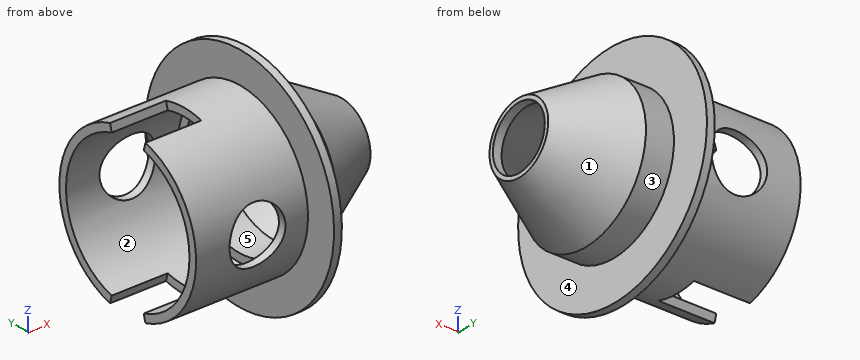
from build123d import *

# Parameters (mm, degrees)
F3_DEPTH = 6.35
F5_D     = 6.35
F6_D     = 6.35


with BuildPart() as f1:
    # F0 (on Front) → F1 (revolve)
    with BuildSketch(Plane.XZ):
        Polygon((-12.185892, 12.7), (-13.074892, 12.7), (-13.074892, 9.1948), (-25.774892, 9.1948), (-25.774892, 8.3058), (-13.074892, 8.3058), (-13.074892, 7.366), (-9.249099, 7.366), (-2.54, 3.4925), (-1.551914, 3.4925), (-1.551914, 3.948557), (-9.010892, 8.255), (-12.185892, 8.255), align=None)
    revolve(axis=Axis((-0.259, 0, 0), (1, 0, 0)))

    # F2 (on face) → F3 (cut)
    with BuildSketch(Plane(origin=(-25.774892, 0, 0), x_dir=(0, -1, 0), z_dir=(-1, 0, 0))):
        with BuildLine():
            Line((2.149699, 8.022787), (2.379789, 8.881495))
            ThreePointArc((2.379789, 8.881495), (0, 9.1948), (-2.379789, 8.881495))
            Line((-2.379789, 8.881495), (-2.149699, 8.022787))
            ThreePointArc((-2.149699, 8.022787), (0, 8.3058), (2.149699, 8.022787))
        make_face()
        with BuildLine():
            Line((-2.149699, -8.022787), (-2.379789, -8.881495))
            ThreePointArc((-2.379789, -8.881495), (0, -9.1948), (2.379789, -8.881495))
            Line((2.379789, -8.881495), (2.149699, -8.022787))
            ThreePointArc((2.149699, -8.022787), (0, -8.3058), (-2.149699, -8.022787))
        make_face()
    extrude(amount=-F3_DEPTH, mode=Mode.SUBTRACT)

    # F5 (through all)
    with Locations(Plane.XZ):
        with Locations((-18.799923, 0)):
            Hole(F5_D / 2)

    # F6 (through all)
    with Locations(Plane(origin=(0, 0, 0), x_dir=(1, 0, 0), z_dir=(0, 1, 0))):
        with Locations((-18.799923, 0)):
            Hole(F6_D / 2)


solid = f1.part
Here's how the part is built. I have some questions about the finished solid (model axes, mm). Face numbers are marked on the shaded views. A direction names the side the tool comes from. Coordinates: 2 decimals unless noted, no trailing zeros. Write each loop counter-clockwise with the first axis right and the second up, starting at its lowest first coordinate (ties: lowest second). Pieces come first, ordered by that corner, then holes.
Item 1: I want a section at D-D on x = -13.5. Write out the boundary of the cut face in (y, z), and give its area (3 significant figures).
Item 2: If we mould it in two halves opening along Y, with no side actions, what happens to the marked faces 3, 4 and 5? For each: +Y half, -Y half, draft (parallel to the pull), parting line (faces both ways), or undercut.
Item 3: I want a section at A-A on z = 0. Count the separate pieces of the cut face and the enclosed holes in it, and give its area (3 significant figures).
Item 4: I want a section at B-B on y = 0. Write out the boundary of the cut face in (x, z) (1 decimal).
Item 5: I want a section at C-C on x = -20.25. Write out the boundary of the cut face in (y, z), and give its area (3 significant figures).
Item 6: If I drill on line 1 (Y direction, x = -10.1, z = 0) (3 decimals); line 2 (X direction, y = 8.45, z = 0); line 3 (Y direction, x = -7, z = -5), over which ranges is the centre line in solid material (lowest first)?
Item 7: On a 3-axis mill with a long thin cutter (end or side, diameter ignored), from which of +Z, -Z, +X, -X, +Y, -Y can I reach the whole of each face in a straight line? I mean the marked faces 1 and 2. Say none if no direction works.
Item 8: Will these pins go through, and if not, where does the flat tip stop? pin 1 (5 mm diameter, centred on y = 4.5, z = 2.5, fed in from -X); pin 2 (8 mm diameter, centred on y = -5, z = 8.5, fed in from +X); pin 3 (8.5 mm diameter, centred on x = -18.8, z = 0, fed in from +Y); pin 4 (5.5 mm diameter, centred on y = 0, z = 0, fed in from +X).
Findings below:
1. outline: circle Ø18.39 at (0, 0); hole circle Ø16.61 at (0, 0)
1. area: 48.9 mm2
2. face 3: parting line
2. face 4: draft
2. face 5: undercut
3. separate pieces: 4
3. enclosed holes: 0
3. area: 41.2 mm2
4. outline: (-19.4, -9.2) - (-13.1, -9.2) - (-13.1, -12.7) - (-12.2, -12.7) - (-12.2, -8.3) - (-9, -8.3) - (-1.6, -3.9) - (-1.6, -3.5) - (-2.5, -3.5) - (-9.2, -7.4) - (-13.1, -7.4) - (-13.1, -8.3) - (-19.4, -8.3) - close; (-19.4, 8.3) - (-13.1, 8.3) - (-13.1, 7.4) - (-9.2, 7.4) - (-2.5, 3.5) - (-1.6, 3.5) - (-1.6, 3.9) - (-9, 8.3) - (-12.2, 8.3) - (-12.2, 12.7) - (-13.1, 12.7) - (-13.1, 9.2) - (-19.4, 9.2) - close
5. outline: (-8.75, -2.82) arc R9.19 ccw to (-2.38, -8.88) - (-2.15, -8.02) arc R8.31 cw to (-7.81, -2.82) - close; (-8.75, 2.82) - (-7.81, 2.82) arc R8.31 cw to (-2.15, 8.02) - (-2.38, 8.88) arc R9.19 ccw to start; (2.15, -8.02) - (2.38, -8.88) arc R9.19 ccw to (8.75, -2.82) - (7.81, -2.82) arc R8.31 cw to start; (2.15, 8.02) arc R8.31 cw to (7.81, 2.82) - (8.75, 2.82) arc R9.19 ccw to (2.38, 8.88) - close
5. area: 30.5 mm2
6. line 1: y = -8.255 to -7.366, 7.366 to 8.255
6. line 2: x = -25.77 to -21.97, -15.62 to -12.19
6. line 3: y = -5.03 to -3.44, 3.44 to 5.03
7. face 1: +X
7. face 2: -X
8. pin 1: stops at x = -13.07
8. pin 2: stops at x = -4.87
8. pin 3: stops at y = 9.19
8. pin 4: passes through
